Can you work these out from the model? Positions are in its coordinate system, mm. Face numbers are marked on the shaded views. Round coordinates to 2 decimals unless told otherwise and drop trailing zeros. Loops run counter-clockwise (first coordinate to the right, second up) from the corner with the lowest first, then second, coordinate; pieces in that order, holes last. Notation, with made-up numbers: (29, 5.25) - (51, 5.25) arc R26 cw to (51, 26.25) - close; hole circle Ø6 at (81.25, 88). An arc over 180 degrees is marked (long way). Answer as CSV lines item,"result".
```python
from build123d import *

# Parameters (mm, degrees)
SKETCH1_W           = 184.15
SKETCH1_H           = 25.4
BOSS_EXTRUDE1_DEPTH = 6.35
SKETCH4_W           = 6.35
SKETCH4_H           = 8.466666667
CUT_EXTRUDE1_DEPTH  = 187.001895152
SKETCH5_W           = 19.05
SKETCH5_H           = 8.466666667
CUT_EXTRUDE2_DEPTH  = 6.35
SKETCH6_W           = 6.35
SKETCH6_H           = 8.466666666
CUT_EXTRUDE3_DEPTH  = 3.175
CHAMFER3_SIZE2      = 3.175
CHAMFER3_SIZE       = 12.7


with BuildPart() as part:
    # Sketch1 → Boss-Extrude1 (new body)
    with BuildSketch(Plane(origin=(0, 0, 0), x_dir=(1, 0, 0), z_dir=(0, 1, 0))):
        with Locations((92.075, -12.7)):
            Rectangle(SKETCH1_W, SKETCH1_H)
    extrude(amount=BOSS_EXTRUDE1_DEPTH)

    # Sketch4 → Cut-Extrude1 (cut, through all)
    with BuildSketch(Plane(origin=(0, 6.35, 0), x_dir=(1, 0, 0), z_dir=(0, 1, 0))):
        with Locations((3.175, -4.233333334)):
            Rectangle(SKETCH4_W, SKETCH4_H)
        with Locations((3.175, -21.166666666)):
            Rectangle(SKETCH4_W, SKETCH4_H)
    extrude(amount=-CUT_EXTRUDE1_DEPTH, mode=Mode.SUBTRACT)

    # Sketch5 → Cut-Extrude2 (cut)
    with BuildSketch(Plane(origin=(0, 6.35, 0), x_dir=(1, 0, 0), z_dir=(0, 1, 0))):
        with Locations((174.625, -21.166666666)):
            Rectangle(SKETCH5_W, SKETCH5_H)
        with Locations((174.625, -4.233333334)):
            Rectangle(SKETCH5_W, SKETCH5_H)
    extrude(amount=-CUT_EXTRUDE2_DEPTH, mode=Mode.SUBTRACT)

    # Sketch6 → Cut-Extrude3 (cut)
    with BuildSketch(Plane.XZ):
        with Locations((168.275, 12.7)):
            Rectangle(SKETCH6_W, SKETCH6_H)
    extrude(amount=-CUT_EXTRUDE3_DEPTH, mode=Mode.SUBTRACT)

    # Chamfer3
    chamfer3_edges = [part.edges().sort_by_distance(p)[0] for p in [
        (184.15, 0, 12.7),
    ]]
    chamfer3_side = [part.faces().sort_by_distance(p)[0] for p in [
        (184.0865, 0, 12.7),
    ]]
    chamfer(chamfer3_edges, length=CHAMFER3_SIZE - 0.0001, length2=CHAMFER3_SIZE2 - 0.0001, reference=chamfer3_side[0])  # a hair under: the kernel refuses the full size


solid = part.part
```
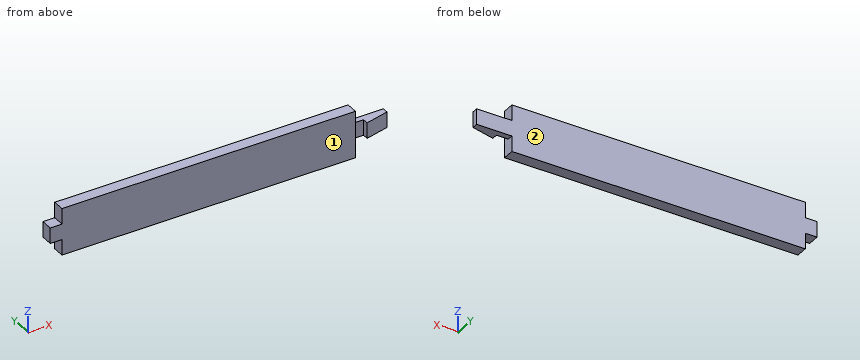
Q1. I'm going to push flat-ended pins straight in: pin 1 Ø1.9 at (y, z) = (4, 6) entering from -X; pin 2 Ø1.9 at (x, y) = (179, 4) entering from -Z; pin 3 Ø1.9 at (x, y) = (173, 4.5) entering from +Z. Where does each tip first touch, or does it pass through?
Checks:
pin 1,"x = 6.35"
pin 2,"z = 8.47"
pin 3,"z = 16.93"
Q2. Imagine slicing it at A-A (y = 1.75). Write out the boundary of the cut face in (x, z), then the cut area to 3 significant figures.
Checks:
outline,"(0, 8.47) - (6.35, 8.47) - (6.35, 0) - (165.1, 0) - (165.1, 25.4) - (6.35, 25.4) - (6.35, 16.93) - (0, 16.93) - close; (171.45, 8.47) - (178.45, 8.47) - (178.45, 16.93) - (171.45, 16.93) - close"
area,"4,150 mm²"
Q3. We'd pull the mould along Y, two halves only. Please class the marked faces 1 and 2: pulls with the +Y half, pulls with the -Y half, needs draft (parallel to the pull), parting line crosses it, or undercut.
Checks:
face 1,"pulls with the -Y half"
face 2,"pulls with the +Y half"
Q4. If I drill on line 1 along X through (y, z) = (2.25, 3.5); line 2 along Y through (x, z) = (172, 10.75), over which ranges is the centre line in solid material (lowest first)? Write a range as [from, to].
Checks:
line 1,"[6.35, 165.1]"
line 2,"[0.14, 6.35]"
